Work out the finished part from the listing and answer in its coordinate system (mm). A direction names the side the tool comes from. Coordinates: 2 decimals unless noted, no trailing zeros. Loops run counter-clockwise (first coordinate to the right, second up) from the corner with the lowest first, then second, coordinate; pieces in that order, holes last. Notation, with made-up numbers: (49.5, -26) - (61.5, -26) arc R17 ccw to (61.5, -14) - close; hole circle Ø4 at (16, 30.5). An arc over 180 degrees is marked (long way). Write each question's results on one line, items separated by ' | '. Start each with the question number.
1. A cutting plane is placed at C-C on y = 38. Determine the outline of the cut face in (x, z).
2. A cutting plane is placed at D-D on z = 14.5. Determine the outline of the cut face in (x, y).
3. Determine the mould class of faces 1 (the cylindrical face through (-9.667, -9.353, 1.269)), 2 (the cylindrical face through (13.887, 24.65, 10.648)), 3 (the flat face through (16, 50, 5)) for opening direction Z: released by +Z, released by -Z, zero draft, split by the parting line, or undercut.
4. A cutting plane is placed at A-A on z = 0. Determine the outline of the cut face in (x, y).
5. Find the intervals of material crossed by line 1 along Z through (x, y) = (0, -12.5); line 2 along Z through (x, y) = (0, 17); line 3 along Y through (x, z) = (-9, 13), in increasing order. Write a range as [from, to].
6. Each of these flat-tipped pins is pushed along its axis until it touches: P1, Ø3, axis at x = 14, y = 3, coming from the +Z side; P2, Ø8, axis at y = 28, z = 11.5, coming from the +X side; P3, Ø6, axis at y = 19, z = 10.5, coming from the -X side; P4, Ø12, axis at x = -13, z = -2.5, coming from the -Y side. Where does it stop, or does it pass through?
7. A cutting plane is placed at B-B on x = 1. Determine the outline of the cut face in (y, z), then the cut area to 3 significant figures.
8. Which of the six approach directions +Z, -Z, +X, -X, +Y, -Y give full straight-line access (tool end or side, diameter ignored) to faces 4 (the cylindrical face through (2.17, -9.86, -9.76)), 5 (the flat face through (-7.1, 1, -7.1))?
Autodesk Inventor part; units mm, degrees
ref_plane "YZ Plane" through (0, 0, 0) normal (1, 0, 0) x (0, 1, 0)
ref_plane "XZ Plane" through (0, 0, 0) normal (0, 1, 0) x (-1, 0, 0)
ref_plane "XY Plane" through (0, 0, 0) normal (0, 0, 1) x (1, 0, 0)
sketch "Sketch1" plane through (0, 0, 0) normal (0, 1, 0) x (-1, 0, 0)
  circle A0 centre (0, 0) radius 17.5
  circle A1 centre (0, 0) radius 10
  dimension "d0" = 35
  dimension "d1" = 20
extrude "Extrusion1" add sketch "Sketch1" along normal blind 50 contours A0 | A1
extrude "Extrusion2" add sketch "Sketch1" against normal blind 20 contours A1
shell "Shell1" thickness 1 removed faces 1 at (-4.3663, 50, -1.0762)
sketch "Sketch2" plane through (0, -20, 0) normal (0, -1, 0) x (1, 0, 0)
  point P0 (0, 0)
  point P1 (0, 0)
hole "Hole1" at (0, -20, 0) direction (0, 1, 0) diameter 19.5 depth 50
properties part number "new seed container"
Values:
1) outline: circle Ø35 at (0, 0); hole circle Ø33 at (0, 0)
2) outline: (-9.8, 0) - (9.8, 0) - (9.8, 50) - (7.87, 50) - (7.87, 1) - (-7.87, 1) - (-7.87, 50) - (-9.8, 50) - close
3) face 1: undercut | face 2: split by the parting line | face 3: zero draft
4) outline: (-17.5, 0) - (-10, 0) - (-10, -20) - (-9.75, -20) - (-9.75, 1) - (-16.5, 1) - (-16.5, 50) - (-17.5, 50) - close; (9.75, -20) - (10, -20) - (10, 0) - (17.5, 0) - (17.5, 50) - (16.5, 50) - (16.5, 1) - (9.75, 1) - close
5) line 1: [-10, -9.75], [9.75, 10] | line 2: [-17.5, -16.5], [16.5, 17.5] | line 3: [0, 1]
6) P1: z = 12.25 | P2: x = 15.81 | P3: x = -15.81 | P4: y = -20
7) outline: (-20, -9.95) - (0, -9.95) - (0, -17.47) - (50, -17.47) - (50, -16.47) - (1, -16.47) - (1, -9.7) - (-20, -9.7) - close; (-20, 9.7) - (1, 9.7) - (1, 16.47) - (50, 16.47) - (50, 17.47) - (0, 17.47) - (0, 9.95) - (-20, 9.95) - close | area: 124 mm^2
8) face 4: -Y | face 5: +Y
